```python
from build123d import *

# Parameters (mm, degrees)
F0_W     = 50
F0_H     = 30
F0_W_2   = 44
F0_H_2   = 24
F1_DEPTH = 341
F2_R     = 1.5
F3_R     = 4.5


with BuildPart() as f1:
    # F0 (on Right) → F1 (new body, symmetric)
    with BuildSketch(Plane.YZ):
        Rectangle(F0_W, F0_H)
        Rectangle(F0_W_2, F0_H_2, mode=Mode.SUBTRACT)
    extrude(amount=F1_DEPTH, both=True)

    # F2
    f2_edges = [f1.edges().sort_by_distance(p)[0] for p in [
        (0, -22, -12),
        (0, -22, 12),
        (0, 22, -12),
        (0, 22, 12),
    ]]
    fillet(f2_edges, radius=F2_R)

    # F3
    f3_edges = [f1.edges().sort_by_distance(p)[0] for p in [
        (0, -25, 15),
        (0, -25, -15),
        (0, 25, -15),
        (0, 25, 15),
    ]]
    fillet(f3_edges, radius=F3_R)


solid = f1.part
```
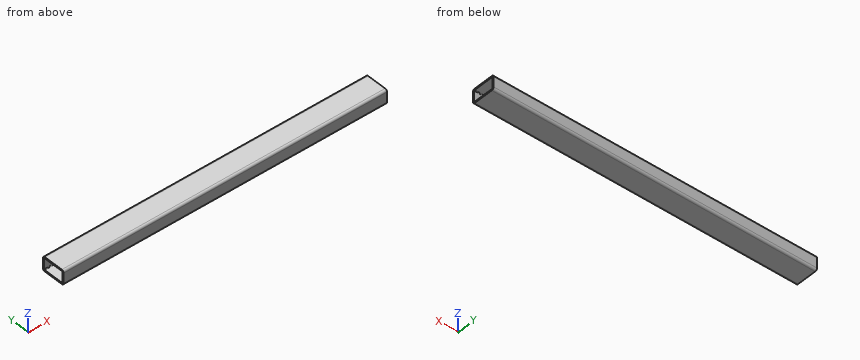
Model file for the job. Use its own axes, mm. Coordinates: 2 decimals unless noted, no trailing zeros. Order: outer loops, then holes, each group sorted by start corner. A loop starts at its lowest first (then second) coordinate and runs counter-clockwise, first axis right, second up. Notation, with made-up numbers: (11.25, 37) -> (19.25, 37) arc R18 cw to (19.25, 52) -> close; hole circle Ø11 at (-29, 47.5). An arc over 180 degrees is marked (long way). Return JSON: item names as keys, results as strings.
Item 1: Slice it at A-A (y = -0.5). Write the cut outline in (x, z), then the cut area to 3 significant figures.
Model answer:
{"outline": "(-341, -15) -> (341, -15) -> (341, -12) -> (-341, -12) -> close; (-341, 12) -> (341, 12) -> (341, 15) -> (-341, 15) -> close", "area": "4,090 mm²"}
Item 2: Wall check: line 1 along Z through (x, y) = (64, 2); line 2 along Y through (x, z) = (181, 10); line 3 along Y through (x, z) = (-301, 13.75). Give the ranges that are in metal, low to high. Write a range as from..to.
Model answer:
{"line 1": "z = -15..-12, 12..15", "line 2": "y = -25..-22, 22..25", "line 3": "y = -23.61..23.61"}
Item 3: Slice it at B-B (z = -4). Write the cut outline in (x, y), then the cut area to 3 significant figures.
Model answer:
{"outline": "(-341, -25) -> (341, -25) -> (341, -22) -> (-341, -22) -> close; (-341, 22) -> (341, 22) -> (341, 25) -> (-341, 25) -> close", "area": "4,090 mm²"}
Item 4: Slice it at C-C (x = 156). Write the cut outline in (y, z), then the cut area to 3 significant figures.
Model answer:
{"outline": "(-25, -10.5) arc R4.5 ccw to (-20.5, -15) -> (20.5, -15) arc R4.5 ccw to (25, -10.5) -> (25, 10.5) arc R4.5 ccw to (20.5, 15) -> (-20.5, 15) arc R4.5 ccw to (-25, 10.5) -> close; hole (-22, -10.5) arc R1.5 ccw to (-20.5, -12) -> (20.5, -12) arc R1.5 ccw to (22, -10.5) -> (22, 10.5) arc R1.5 ccw to (20.5, 12) -> (-20.5, 12) arc R1.5 ccw to (-22, 10.5) -> close", "area": "429 mm²"}
